Design review of the part built by this model. Coordinates are the model's own, in mm. Coordinates: 2 decimals unless noted, no trailing zeros. Write each loop counter-clockwise with the first axis right and the second up, starting at its lowest first coordinate (ties: lowest second). Pieces come first, ordered by that corner, then holes.
Q1. Take a section at C-C (z = -1.55). State how many separate pieces and enclosed holes the cut face has, and give its area (3 significant figures).
Q2. Take a section at D-D (x = 25). Give the boundary of the cut face in (y, z).
Q3. For probe 1 along X at (y, z) = (10, -0.4); probe 2 along X at (y, z) = (0.5, -2.2); probe 3 along Y at (x, z) = (-110, -3.55), list the stretches that pass through material, from the lowest coordinate up.
Q4. Take a section at B-B (y = 0). Give the boundary of the cut face in (x, z).
Q5. Take a section at A-A (x = 100). Give the boundary of the cut face in (y, z).
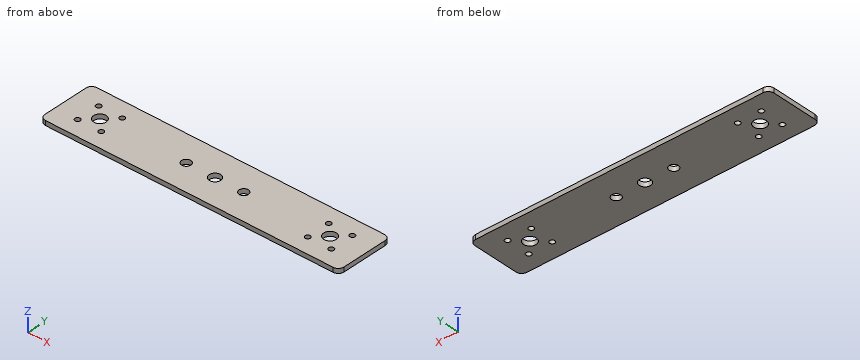
```python
from build123d import *

# Parameters (mm, degrees)
SKETCH1_W          = 260
SKETCH1_H          = 50
BASE_FLANGE1_DEPTH = 4
SKETCH6_R          = 5.5
SKETCH6_R_2        = 5
SKETCH6_R_3        = 4
SKETCH6_R_4        = 2.25
CUT_EXTRUDE1_DEPTH = 10
FILLET1_R          = 5


# Sheet-metal steps are written as plain solids
with BuildPart() as part:
    # Sketch1 → Base-Flange1 (new body)
    with BuildSketch(Plane.XY):
        Rectangle(SKETCH1_W, SKETCH1_H)
    extrude(amount=-BASE_FLANGE1_DEPTH)

    # Sketch6 → Cut-Extrude1 (cut)
    with BuildSketch(Plane.XY):
        with Locations((100, 0)):
            Circle(SKETCH6_R)
        with Locations((-100, 0)):
            Circle(SKETCH6_R)
        Circle(SKETCH6_R_2)
        with Locations((-25, 0)):
            Circle(SKETCH6_R_3)
        with Locations(Location((25, 0, 0), (0, 0, 180))):
            Circle(SKETCH6_R_3)
        with Locations((110.253048327, 10.253048327)):
            Circle(SKETCH6_R_4)
        with Locations(Location((89.746951673, 10.253048327, 0), (0, 0, 180))):
            Circle(SKETCH6_R_4)
        with Locations((89.746951673, -10.253048327)):
            Circle(SKETCH6_R_4)
        with Locations(Location((110.253048327, -10.253048327, 0), (0, 0, 180))):
            Circle(SKETCH6_R_4)
        with Locations((-110.253048327, -10.253048327)):
            Circle(SKETCH6_R_4)
        with Locations(Location((-89.746951673, -10.253048327, 0), (0, 0, 180))):
            Circle(SKETCH6_R_4)
        with Locations((-89.746951673, 10.253048327)):
            Circle(SKETCH6_R_4)
        with Locations(Location((-110.253048327, 10.253048327, 0), (0, 0, 180))):
            Circle(SKETCH6_R_4)
    extrude(amount=-CUT_EXTRUDE1_DEPTH, mode=Mode.SUBTRACT)

    # Fillet1
    fillet1_edges = [part.edges().sort_by_distance(p)[0] for p in [
        (130, -25, -2),
        (-130, -25, -2),
        (-130, 25, -2),
        (130, 25, -2),
    ]]
    fillet(fillet1_edges, radius=FILLET1_R)


solid = part.part
```
Response:
1. separate pieces: 1
1. enclosed holes: 13
1. area: 12,500 mm2
2. outline: (-25, -4) - (-4, -4) - (-4, 0) - (-25, 0) - close; (4, -4) - (25, -4) - (25, 0) - (4, 0) - close
3. probe 1: x = -130 to -112.49, -108.02 to -91.98, -87.51 to 87.51, 91.98 to 108.02, 112.49 to 130
3. probe 2: x = -130 to -105.48, -94.52 to -28.97, -21.03 to -4.97, 4.97 to 21.03, 28.97 to 94.52, 105.48 to 130
3. probe 3: y = -25 to -12.49, -8.02 to 8.02, 12.49 to 25
4. outline: (-130, -4) - (-105.5, -4) - (-105.5, 0) - (-130, 0) - close; (-94.5, -4) - (-29, -4) - (-29, 0) - (-94.5, 0) - close; (-21, -4) - (-5, -4) - (-5, 0) - (-21, 0) - close; (5, -4) - (21, -4) - (21, 0) - (5, 0) - close; (29, -4) - (94.5, -4) - (94.5, 0) - (29, 0) - close; (105.5, -4) - (130, -4) - (130, 0) - (105.5, 0) - close
5. outline: (-25, -4) - (-5.5, -4) - (-5.5, 0) - (-25, 0) - close; (5.5, -4) - (25, -4) - (25, 0) - (5.5, 0) - close
